Geometry: see drawing. Coordinates: mm, zero at the bounding-box minimum. Round coordinates to 2 decimals unless told otherwise and drop trailing zeros. Loops run counter-clockwise (first coordinate to the right, second up) from the corner with the lowest first, then second, coordinate; pieces in that order, holes last. Notation, with made-up numbers: (39, 15) -> (64, 15) arc R29 cw to (64, 53) -> close; hole circle Ø11 at (47.25, 50). An arc over 180 degrees is marked (long way). Write item = value, one per line.
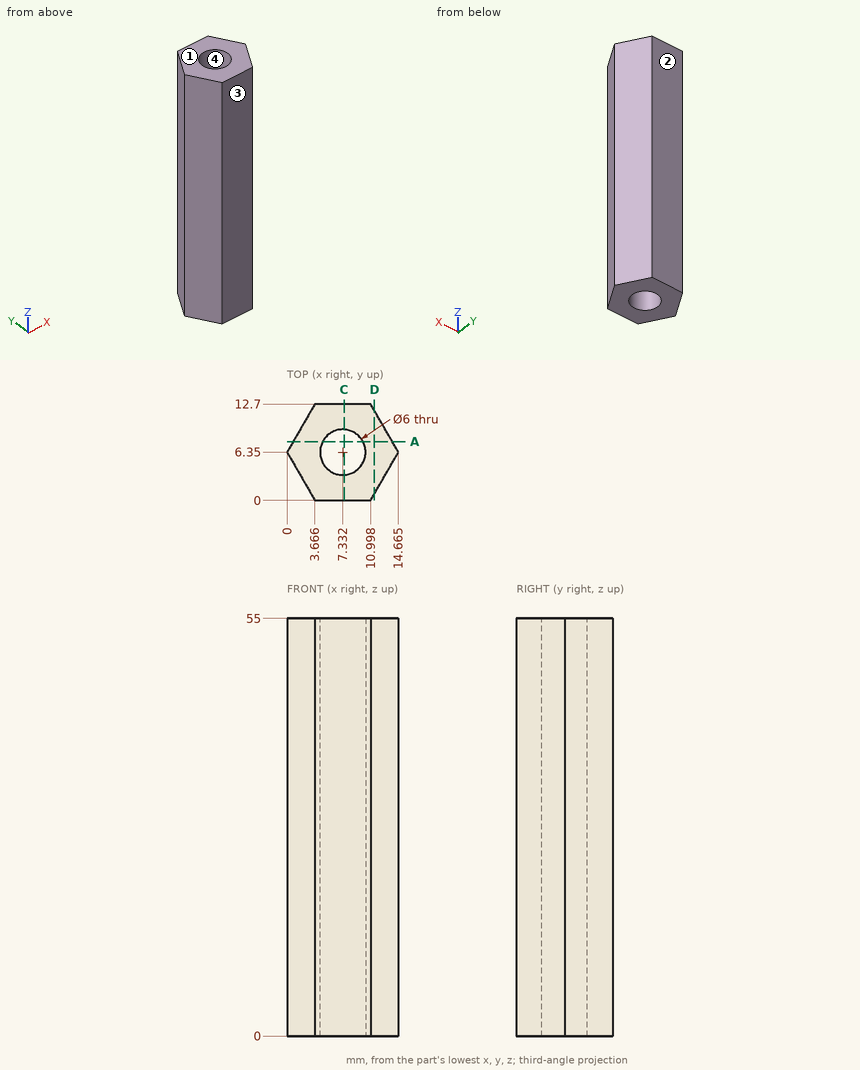
1. Section query A-A (y = 7.75). Return the cut outline in (x, z) (1 decimal).
Evaluation:
outline = (0.8, 0) -> (4.7, 0) -> (4.7, 55) -> (0.8, 55) -> close; (10, 0) -> (13.9, 0) -> (13.9, 55) -> (10, 55) -> close
2. Section query C-C (x = 7.5). Return the cut outline in (y, z) (1 decimal), then the cut area to 3 significant figures.
Evaluation:
outline = (0, 0) -> (3.4, 0) -> (3.4, 55) -> (0, 55) -> close; (9.3, 0) -> (12.7, 0) -> (12.7, 55) -> (9.3, 55) -> close
area = 369 mm²
3. Section query D-D (x = 11.5). Return the cut outline in (y, z), then the cut area to 3 significant figures.
Evaluation:
outline = (0.87, 0) -> (11.83, 0) -> (11.83, 55) -> (0.87, 55) -> close
area = 603 mm²
4. Line query: probe 1 along Y at (x, z) = (7.5, 13.5) (1 decimal); probe 2 along X at (y, z) = (7.25, 4) (1 decimal); probe 3 along X at (y, z) = (5.5, 47.5) (1 decimal). Output: solid intervals per line, ascending. Write a range as from..to.
Evaluation:
probe_1 = 0..3.4, 9.3..12.7
probe_2 = 0.5..4.5, 10.2..14.1
probe_3 = 0.5..4.5, 10.2..14.2
5. Contact query for flat-ended pins moving along their axis: pin 1 Ø6 at (y, z) = (7, 29.5) entering from +X (1 decimal); pin 2 Ø2 at (x, z) = (2.5, 46) entering from -Y (1 decimal); pin 3 Ø5 at (y, z) = (7, 42) entering from -X. Output: stop coordinate, or through.
Evaluation:
pin_1 = 14.7
pin_2 = 0.3
pin_3 = 0
6. Mould query, pull axis Y, two halves, no side actions, for the marked faces 1, 2, 3 and 4. Classes: released by +Y, released by -Y, zero draft, split by the parting line, or undercut.
Evaluation:
face_1 = zero draft
face_2 = released by +Y
face_3 = released by -Y
face_4 = undercut
